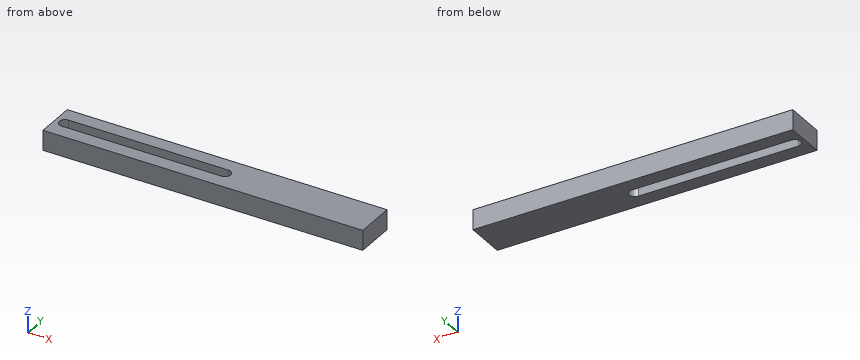
```python
from build123d import *

# Parameters (mm, degrees)
SKETCH1_W               = 203.2
SKETCH1_H               = 25.4
BOSS_EXTRUDE1_DEPTH     = 6.35
CUT_EXTRUDE1_DEPTH      = 104.175287739
CUT_EXTRUDE1_DEPTH_BACK = 104.175287739


with BuildPart() as part:
    # Sketch1 → Boss-Extrude1 (new, symmetric)
    with BuildSketch(Plane.XY):
        Rectangle(SKETCH1_W, SKETCH1_H)
    extrude(amount=BOSS_EXTRUDE1_DEPTH, both=True)

    # Sketch2 → Cut-Extrude1 (cut, two sides: drawn at the far end of the back side and taken through both)
    with BuildSketch(Plane.XY.offset(6.35).offset(-CUT_EXTRUDE1_DEPTH_BACK)):
        with BuildLine():
            Line((-95.25, 3.675), (6.35, 3.675))
            ThreePointArc((6.35, 3.675), (10.025, 0), (6.35, -3.675))
            Line((6.35, -3.675), (-95.25, -3.675))
            ThreePointArc((-95.25, -3.675), (-98.925, 0), (-95.25, 3.675))
        make_face()
    extrude(amount=CUT_EXTRUDE1_DEPTH + CUT_EXTRUDE1_DEPTH_BACK, mode=Mode.SUBTRACT)


solid = part.part
```
Model file for the job. Use its own axes, mm. Coordinates: 2 decimals unless noted, no trailing zeros. Loops run counter-clockwise (first coordinate to the right, second up) from the corner with the lowest first, then second, coordinate; pieces in that order, holes last. Notation, with made-up numbers: M 68,-11 L 108,-11 A31 cw 108,16 Z; hole C -7.5,49 d7. An arc over 180 degrees is marked long. Use CSV: the item, a comma, the result in double quotes. Start each with the question number.
1. Band-saw the part on B-B, the plane z = -3. List the corners of the cut face in (x, y) (3 decimals), then the cut area to 3 significant figures.
2. Band-saw the part on A-A, the plane x = -9. List the corners of the cut face in (y, z) (3 decimals), then the cut area to 3 significant figures.
3. Probe probe 1 along Y at (x, z) = (-65.5, 4.5) (3 decimals); probe 2 along X at (y, z) = (1.75, 5.5); probe 3 along X at (y, z) = (1.25, -5). List the from-to ranges inside material, lowest first. Write a range as [from, to].
4. Band-saw the part on C-C, the plane y = 0. List the corners of the cut face in (x, z) (3 decimals).
Entries:
1,outline,"M -101.6,-12.7 L 101.6,-12.7 L 101.6,12.7 L -101.6,12.7 Z; hole M -95.25,-3.675 L 6.35,-3.675 A3.675 ccw 6.35,3.675 L -95.25,3.675 A3.675 ccw Z"
1,area,"4,370 mm2"
2,outline,"M -12.7,-6.35 L -3.675,-6.35 L -3.675,6.35 L -12.7,6.35 Z; M 3.675,-6.35 L 12.7,-6.35 L 12.7,6.35 L 3.675,6.35 Z"
2,area,"229 mm2"
3,probe 1,"y = [-12.7, -3.675], [3.675, 12.7]"
3,probe 2,"x = [-101.6, -98.48], [9.58, 101.6]"
3,probe 3,"x = [-101.6, -98.71], [9.81, 101.6]"
4,outline,"M -101.6,-6.35 L -98.925,-6.35 L -98.925,6.35 L -101.6,6.35 Z; M 10.025,-6.35 L 101.6,-6.35 L 101.6,6.35 L 10.025,6.35 Z"
